```python
from build123d import *
from build123d.topology import SkipClean

# Parameters (mm, degrees)
SKETCH_2_W           = 98
SKETCH_2_H           = 78
SKETCH_2_R           = 2.25
EXTRUDE_1_DEPTH      = 25
SKETCH_4_W           = 94.182021657
SKETCH_4_H           = 15.686226028
CUT_EXTRUDE_1_DEPTH  = 15
CUT_EXTRUDE_START    = -21.5
SKETCH_3_W           = 94
SKETCH_3_H           = 70
SKETCH_3_R           = 2.25
CUT_EXTRUDE_2_DEPTH  = 18.5
CUT_EXTRUDE_3_REACH  = 74.064
SKETCH_5_R           = 4
EXTRUDE_3_DEPTH      = 22
EXTRUDE_3_DEPTH_BACK = 3
SKETCH_6_W           = 11.966924864
SKETCH_6_H           = 10.472950633
SKETCH_6_R           = 2
SKETCH_6_W_2         = 10.715562549
SKETCH_6_H_2         = 10.536387569
SKETCH_7_R           = 3
CUT_EXTRUDE_4_DEPTH  = 15
SKETCH_9_W           = 94
SKETCH_9_H           = 18.5
CUT_EXTRUDE_5_DEPTH  = 15
EXTRUDE_START        = 2.5
SKETCH_10_R          = 4
SKETCH_10_R_2        = 2.25
EXTRUDE_4_DEPTH      = 2.5
FILLET_1_R           = 10
SKETCH_12_R          = 1.75
CUT_EXTRUDE_6_DEPTH  = 111.498829227
CUT_EXTRUDE_7_DEPTH  = 2.6


with BuildPart() as part:
    # 草图2 → 凸台-拉伸1 (new body)
    with BuildSketch(Plane.XY):
        with Locations((2.33490566, 4.964622642)):
            Rectangle(SKETCH_2_W, SKETCH_2_H)
        with Locations((-20.66509434, 26.964622642)):
            Circle(SKETCH_2_R, mode=Mode.SUBTRACT)
        with Locations((25.33490566, 26.964622642)):
            Circle(SKETCH_2_R, mode=Mode.SUBTRACT)
    extrude(amount=EXTRUDE_1_DEPTH)

    # 草图4 → 切除-拉伸1 (cut)
    with BuildSketch(Plane.XZ.offset(34.035377358)):
        with Locations((2.785262667, 9.306899291)):
            Rectangle(SKETCH_4_W, SKETCH_4_H)
    extrude(amount=-CUT_EXTRUDE_1_DEPTH, mode=Mode.SUBTRACT)

    # 草图3 → 切除-拉伸2 (cut)
    with BuildSketch(Plane.XY.offset(25).offset(CUT_EXTRUDE_START)):
        with Locations((2.33490566, 4.964622642)):
            Rectangle(SKETCH_3_W, SKETCH_3_H)
        with Locations((-20.66509434, 26.964622642)):
            Circle(SKETCH_3_R, mode=Mode.SUBTRACT)
        with Locations((25.33490566, 26.964622642)):
            Circle(SKETCH_3_R, mode=Mode.SUBTRACT)
    extrude(amount=CUT_EXTRUDE_2_DEPTH, mode=Mode.SUBTRACT)

    # 草图5 → 切除-拉伸3 (cut, up to next)
    with BuildSketch(Plane(origin=(0, 0, 0), x_dir=(-1, 0, 0), z_dir=(0, 0, -1)), mode=Mode.PRIVATE) as cut_extrude_3_sk1:
        with Locations((-25.33490566, 26.964622642)):
            Circle(SKETCH_5_R)
    cut_extrude_3_tool1 = extrude(cut_extrude_3_sk1.sketch, amount=-CUT_EXTRUDE_3_REACH, mode=Mode.PRIVATE) & part.part
    # 草图5 → 切除-拉伸3 (cut, up to next)
    with BuildSketch(Plane(origin=(0, 0, 0), x_dir=(-1, 0, 0), z_dir=(0, 0, -1)), mode=Mode.PRIVATE) as cut_extrude_3_sk2:
        with Locations((20.66509434, 26.964622642)):
            Circle(SKETCH_5_R)
    cut_extrude_3_tool2 = extrude(cut_extrude_3_sk2.sketch, amount=-CUT_EXTRUDE_3_REACH, mode=Mode.PRIVATE) & part.part
    add(cut_extrude_3_tool1.solids().sort_by_distance((25.334906, 26.964623, 0))[0], mode=Mode.SUBTRACT)
    add(cut_extrude_3_tool2.solids().sort_by_distance((-20.665094, 26.964623, 0))[0], mode=Mode.SUBTRACT)

    # 草图6 → 凸台-拉伸3 (add, two sides: drawn at the far end of the back side and taken through both)
    # profile 1 of 2: a face of its own
    with BuildSketch(Plane(origin=(0, 0, 22), x_dir=(-1, 0, 0), z_dir=(0, 0, -1)).offset(-EXTRUDE_3_DEPTH_BACK)):
        with Locations((40.681631908, -39.271852675)):
            Rectangle(SKETCH_6_W, SKETCH_6_H)
        with Locations((41.16509434, -39.449232705)):
            Circle(SKETCH_6_R, mode=Mode.SUBTRACT)
    # profile 2 of 2: a face of its own
    with BuildSketch(Plane(origin=(0, 0, 22), x_dir=(-1, 0, 0), z_dir=(0, 0, -1)).offset(-EXTRUDE_3_DEPTH_BACK)):
        with Locations((-45.977124386, -39.240134207)):
            Rectangle(SKETCH_6_W_2, SKETCH_6_H_2)
        with Locations((-45.83490566, -39.449232705)):
            Circle(SKETCH_6_R, mode=Mode.SUBTRACT)
    extrude(amount=EXTRUDE_3_DEPTH + EXTRUDE_3_DEPTH_BACK)

    # 草图7 → 切除-拉伸4 (cut)
    with BuildSketch(Plane(origin=(0, 0, 0), x_dir=(-1, 0, 0), z_dir=(0, 0, -1))):
        with Locations((-45.83490566, -39.449232705)):
            Circle(SKETCH_7_R)
        with Locations((41.16509434, -39.449232705)):
            Circle(SKETCH_7_R)
    extrude(amount=-CUT_EXTRUDE_4_DEPTH, mode=Mode.SUBTRACT)

    # 草图9 → 切除-拉伸5 (cut)
    with BuildSketch(Plane.XZ.offset(-39.964622642)):
        with Locations((2.33490566, 12.75)):
            Rectangle(SKETCH_9_W, SKETCH_9_H)
    extrude(amount=-CUT_EXTRUDE_5_DEPTH, mode=Mode.SUBTRACT)

    # 草图10 → 凸台-拉伸4 (add)
    # profile 1 of 2: a face of its own
    with SkipClean():  # the faces are left unmerged after this step: merging them gives an invalid solid
        with BuildSketch(Plane(origin=(0, 0, 22), x_dir=(-1, 0, 0), z_dir=(0, 0, -1)).offset(EXTRUDE_START)):
            with Locations((-25.33490566, 26.964622642)):
                Circle(SKETCH_10_R)
            with Locations((-25.33490566, 26.964622642)):
                Circle(SKETCH_10_R_2, mode=Mode.SUBTRACT)
        # profile 2 of 2: a face of its own
        with BuildSketch(Plane(origin=(0, 0, 22), x_dir=(-1, 0, 0), z_dir=(0, 0, -1)).offset(EXTRUDE_START)):
            with Locations((20.66509434, 26.964622642)):
                Circle(SKETCH_10_R)
            with Locations((20.66509434, 26.964622642)):
                Circle(SKETCH_10_R_2, mode=Mode.SUBTRACT)
        extrude(amount=-EXTRUDE_4_DEPTH)

    # 圆角1
    # the kernel refuses this fillet: 10 mm, written as the material it adds along each edge
    with BuildSketch(Plane(origin=(25.33490566, 26.964622642, 22), x_dir=(-1, 0, 0), z_dir=(0, -1, 0))) as fillet_1_piece_1:
        with BuildLine():
            CenterArc((10.614378278, 10), FILLET_1_R, 228.590377891, 41.409622109)
            Line((4, 2.5), (3.867712434, 2.35))
            ThreePointArc((3.867712434, 2.35), (3.8, 1.25), (3.8, 0))
            Line((3.8, 0), (4, -0.2))
            Line((4, -0.2), (10.614378278, -0.2))
            Line((10.614378278, -0.2), (10.614378278, 0))
        make_face()
    revolve(axis=Axis((25.33490566, 26.964622642, 22), (0, 0, -1)))
    with BuildSketch(Plane(origin=(-20.66509434, 26.964622642, 22), x_dir=(-1, 0, 0), z_dir=(0, -1, 0))) as fillet_1_piece_2:
        with BuildLine():
            CenterArc((10.614378278, 10), FILLET_1_R, 228.590377891, 41.409622109)
            Line((4, 2.5), (3.867712434, 2.35))
            ThreePointArc((3.867712434, 2.35), (3.8, 1.25), (3.8, 0))
            Line((3.8, 0), (4, -0.2))
            Line((4, -0.2), (10.614378278, -0.2))
            Line((10.614378278, -0.2), (10.614378278, 0))
        make_face()
    revolve(axis=Axis((-20.66509434, 26.964622642, 22), (0, 0, -1)))

    # 草图12 → 切除-拉伸6 (cut, through all)
    with BuildSketch(Plane.ZY.offset(46.66509434)):
        with Locations((10.372747463, -23.946592615)):
            Circle(SKETCH_12_R)
        with Locations((12.5, 25.053407385)):
            Circle(SKETCH_12_R)
    extrude(amount=-CUT_EXTRUDE_6_DEPTH, mode=Mode.SUBTRACT)

    # 草图13 → 切除-拉伸7 (cut)
    with BuildSketch(Plane.XY.offset(25)):
        Polygon((-20.66509434, 30.197784149), (-23.46509434, 28.581203395), (-23.46509434, 25.348041888), (-20.66509434, 23.731461134), (-17.86509434, 25.348041888), (-17.86509434, 28.581203395), align=None)
        Polygon((25.33490566, 30.197784149), (22.53490566, 28.581203395), (22.53490566, 25.348041888), (25.33490566, 23.731461134), (28.13490566, 25.348041888), (28.13490566, 28.581203395), align=None)
    extrude(amount=-CUT_EXTRUDE_7_DEPTH, mode=Mode.SUBTRACT)


solid = part.part
```
Geometry check sheet. Reference: the model listing, model coordinates, mm. A direction names the side the tool comes from. Give positions to 0.01 mm unless a question says otherwise; leave off trailing zeros. Order: outer loops, then holes, each group sorted by start corner. A loop starts at its lowest first (then second) coordinate and runs counter-clockwise, first axis right, second up. Notation, with made-up numbers: (76, 42.5) - (89, 42.5) arc R25 ccw to (89, 60.5) - close; hole circle Ø1 at (-37.5, 64.5). An arc over 180 degrees is marked (long way). Answer in a Markdown table with one row per item. Add a question column.
Q1. Tool access check on faces 5 (the flat face through (26.75, 29.38, 23.72)), 6 (the cylindrical face through (28.28, 29.67, 1.73)), 7 (the flat face through (2, -30.035, 19)), 8 (the flat face through (49.335, 6, 13)). Record the directions out of +Z, -Z, +X, -X, +Y, -Y that give a thin tool (end or side, any length) a straight path to the whole face; none if there is none.
Q2. Cross-section at C-C, the plane z = 7.5. Enter the section's corners in (x, y).
Q3. Cross-section at B-B, the plane y = 0. Enter the section's corners in (x, z).
Q4. Material ranges on probe 1 along Z at (x, y) = (12.5, 21); probe 2 along Z at (x, y) = (-38.5, -34); probe 3 along X at (y, z) = (-2, 13), recorded low to high. Write a range as from..to.
Q5. Cross-section at A-A, the plane x = 0. Enter the section's corners in (y, z), then the cut area to 3 significant figures.
Q6. Gauge pin test, flat ends, axial feed: pin 1 (1.8 mm diameter, centred on x = -42, y = -38.5, fed in from -Z); pin 2 (6 mm diameter, centred on x = -20.67, y = 26.96, fed in from -Z); pin 3 (6 mm diameter, centred on x = 32.5, z = 21, fed in from -Y). Record the tip position at first contact, or that the pin passes through.
Q7. Mould release check, pull along Y, two halves, no side actions. Record for faces 1 (the flat face through (-41, -44.508, 13)), 2 (the flat face through (-44.665, 6, 13)), 3 (the flat face through (23.92, 24.55, 23.72)), 4 (the cylindrical face through (-39.58, -40.67, 20.07)): pulls with the +Y half, pulls with the -Y half, needs draft (parallel to the pull), parting line crosses it, or undercut.
Check values:
| question | item | result |
|---|---|---|
| 1 | face 5 | +Z |
| 1 | face 6 | -Z |
| 1 | face 7 | none |
| 1 | face 8 | +Y |
| 2 | outline | (-46.67, -44.51) - (-34.7, -44.51) - (-34.7, -34.04) - (-44.31, -34.04) - (-44.31, -30.04) - (-44.67, -30.04) - (-44.67, 43.96) - (-46.67, 43.96) - close; (40.62, -44.51) - (51.33, -44.51) - (51.33, 43.96) - (49.33, 43.96) - (49.33, -19.04) - (49.88, -19.04) - (49.88, -33.97) - (40.62, -33.97) - close; hole circle Ø6 at (-41.17, -39.45); hole circle Ø6 at (45.83, -39.45) |
| 3 | outline | (-46.67, 0) - (51.33, 0) - (51.33, 25) - (-46.67, 25) - close; hole (-44.67, 3.5) - (49.33, 3.5) - (49.33, 22) - (-44.67, 22) - close |
| 4 | probe 1 | z = 0..3.5, 22..25 |
| 4 | probe 2 | z = 0..1.46, 17.15..25 |
| 4 | probe 3 | x = -46.67..-44.67, 49.33..51.33 |
| 5 | outline | (-34.04, 0) - (43.96, 0) - (43.96, 3.5) - (-19.04, 3.5) - (-19.04, 1.46) - (-34.04, 1.46) - close; (-34.04, 17.15) - (-30.04, 17.15) - (-30.04, 22) - (43.96, 22) - (43.96, 25) - (-34.04, 25) - close |
| 5 | area | 496 mm^2 |
| 6 | pin 1 | stops at z = 15 |
| 6 | pin 2 | stops at z = 19.5 |
| 6 | pin 3 | stops at y = -34.04 |
| 7 | face 1 | pulls with the -Y half |
| 7 | face 2 | needs draft |
| 7 | face 3 | undercut |
| 7 | face 4 | undercut |
